Read the model definition and answer for the solid it produces. Units are mm, in the model's axes. Face numbers are marked on the shaded views. A direction names the side the tool comes from. Round coordinates to 2 decimals unless told otherwise and drop trailing zeros. Order: outer loops, then holes, each group sorted by start corner. A loop starts at its lowest first (then second) coordinate and runs counter-clockwise, first axis right, second up. Notation, with made-up numbers: (21.5, 50) - (59.5, 50) arc R11 cw to (59.5, 55) - close; hole circle Ø7 at (-2.5, 65.5). An arc over 180 degrees is marked (long way). Answer as a JSON object with one key per item and string values. Group by question number.
Q1. Consider line 1 (X direction, y = -48.5, z = 4.5); line 2 (X direction, y = -39, z = 28); line 3 (Z direction, x = 16, y = -14). Determine where each line is inside the solid, lowest interval first.
Q2. The mould has two halves that part along Y. Classify the marked faces 5, 6, 7 and 8: pulls with the +Y half, pulls with the -Y half, needs draft (parallel to the pull), parting line crosses it, or undercut.
Q3. A cutting plane is placed at D-D on x = 56.5. Determine the outline of the cut face in (y, z).
Q4. Given pin 1 Ø15 at (y, z) = (-43.5, 11) entering from -X; pin 2 Ø7.5 at (x, y) = (141.5, -68.5) entering from +Z; pin 3 Ø4 at (y, z) = (-34.5, 20.5) entering from -X, each flat-ended and moving along its own axis, determine where each tip first touches the part or whether it passes through.
Q5. A tool of negligible diameter and unlimited length cuts with its end or side. For the marked faces 1, 2, 3 and 4, from which of +Z, -Z, +X, -X, +Y, -Y can it reach the whole face along a straight path? Write none if from no direction.
Q6. A cutting plane is placed at B-B on x = 19. Determine the outline of the cut face in (y, z), and give its area (3 significant figures).
Q7. A cutting plane is placed at A-A on z = 46.5. Determine the outline of the cut face in (x, y).
Q8. A cutting plane is placed at C-C on y = -9. Determine the outline of the cut face in (x, z), and give its area (3 significant figures).
```python
from build123d import *

# Parameters (mm, degrees)
F1_DEPTH = 76.2
F3_DEPTH = 25.4
F5_DEPTH = 25.4
F7_DEPTH = 101.6


with BuildPart() as f1:
    # F0 (on Front) → F1 (new body)
    with BuildSketch(Plane.XZ):
        Polygon((0, 12.7), (0, 0), (38.1, 0), (38.1, 19.05), (114.3, 19.05), (114.3, 0), (152.4, 0), (152.4, 12.7), (127, 12.7), (127, 50.8), (25.4, 50.8), (25.4, 12.7), align=None)
    extrude(amount=F1_DEPTH)

    # F2 (on face) → F3 (cut)
    with BuildSketch(Plane.XY.offset(12.7)):
        Polygon((127, -25.4), (127, -50.8), (152.4, -76.2), (152.4, 0), align=None)
    extrude(amount=-F3_DEPTH, mode=Mode.SUBTRACT)

    # F4 (on face) → F5 (cut)
    with BuildSketch(Plane.XY.offset(12.7)):
        Polygon((0, -76.2), (25.4, -50.8), (25.4, -25.4), (0, 0), align=None)
    extrude(amount=-F5_DEPTH, mode=Mode.SUBTRACT)

    # F6 (on face) → F7 (cut)
    with BuildSketch(Plane.YZ.offset(127)):
        Polygon((-25.4, 50.8), (-50.8, 50.8), (-38.1, 38.1), align=None)
    extrude(amount=-F7_DEPTH, mode=Mode.SUBTRACT)


solid = f1.part
```
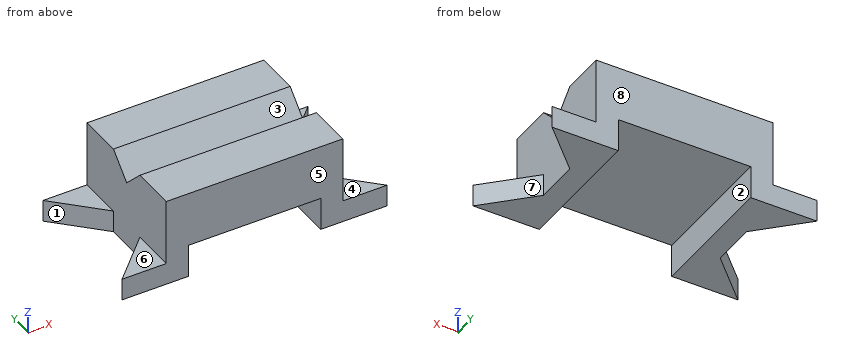
Result set:
{
 "1": {"line 1": "x = 25.4 to 38.1, 114.3 to 127", "line 2": "x = 25.4 to 127", "line 3": "z = 0 to 12.7"},
 "2": {"face 5": "pulls with the -Y half", "face 6": "needs draft", "face 7": "undercut", "face 8": "pulls with the +Y half"},
 "3": {"outline": "(-76.2, 19.05) - (0, 19.05) - (0, 50.8) - (-25.4, 50.8) - (-38.1, 38.1) - (-50.8, 50.8) - (-76.2, 50.8) - close"},
 "4": {"pin 1": "stops at x = 25.2", "pin 2": "stops at z = 12.7", "pin 3": "stops at x = 25.4"},
 "5": {"face 1": "+Z, -Z, -X", "face 2": "-Z, +Y, -Y", "face 3": "+Z, +X, -X", "face 4": "+Z, +X, +Y, -Y"},
 "6": {"outline": "(-76.2, 0) - (-57.2, 0) - (-57.2, 12.7) - (-76.2, 12.7) - close; (-19, 0) - (0, 0) - (0, 12.7) - (-19, 12.7) - close", "area": "483 mm²"},
 "7": {"outline": "(25.4, -76.2) - (127, -76.2) - (127, -46.5) - (25.4, -46.5) - close; (25.4, -29.7) - (127, -29.7) - (127, 0) - (25.4, 0) - close"},
 "8": {"outline": "(9, 0) - (38.1, 0) - (38.1, 19.05) - (114.3, 19.05) - (114.3, 0) - (143.4, 0) - (143.4, 12.7) - (127, 12.7) - (127, 50.8) - (25.4, 50.8) - (25.4, 12.7) - (9, 12.7) - close", "area": "4,130 mm²"}
}
